Build history of the part. All positions in model axes, mm. A direction names the side the tool comes from. Give positions to 0.01 mm unless a question says otherwise; leave off trailing zeros. Write each loop counter-clockwise with the first axis right and the second up, starting at its lowest first coordinate (ties: lowest second). Pieces come first, ordered by that corner, then holes. Notation, with made-up numbers: (43, -24.75) - (77, -24.75) arc R22 ccw to (77, -18.75) - close; hole circle Ø7 at (27, 63). An arc over 180 degrees is marked (long way). Use one line per item in the form item = value. Start each with the question number.
from build123d import *

# Parameters (mm, degrees)
BOSS_EXTRUDE1_DEPTH     = 25.4
SKETCH2_W               = 52
SKETCH2_H               = 63.5
CUT_EXTRUDE1_DEPTH      = 3.175
SKETCH3_W               = 25.4
SKETCH3_H               = 63.5
CUT_EXTRUDE2_DEPTH      = 3.175
SKETCH4_W               = 52
SKETCH4_H               = 63.5
CUT_EXTRUDE3_DEPTH      = 3.175
SKETCH5_W               = 25.4
SKETCH5_H               = 63.5
CUT_EXTRUDE4_DEPTH      = 3.175
SKETCH6_R               = 2.5527
CUT_EXTRUDE5_DEPTH      = 23.225
SKETCH7_R               = 2.5527
CUT_EXTRUDE6_DEPTH      = 150.825
SKETCH8_W               = 101
SKETCH8_H               = 177.8
CUT_EXTRUDE7_DEPTH      = 26.4
CUT_EXTRUDE8_DEPTH      = 1
CUT_EXTRUDE8_DEPTH_BACK = 26.4
CUT_EXTRUDE9_DEPTH      = 26.4
CUT_EXTRUDE10_DEPTH     = 26.4
BOSS_EXTRUDE2_DEPTH     = 25.4
CUT_EXTRUDE11_DEPTH     = 51.8
CUT_EXTRUDE12_DEPTH     = 51.8
CUT_EXTRUDE13_DEPTH     = 93.323036631
CUT_EXTRUDE14_DEPTH     = 51.8
CUT_EXTRUDE15_DEPTH     = 26.4
CUT_EXTRUDE16_DEPTH     = 51.8


with BuildPart() as part:
    # Sketch1 → Boss-Extrude1 (new body)
    with BuildSketch(Plane.XY):
        Polygon((0, 0), (0, 76.2), (-101, 76.2), (-101, 254), (153, 254), (153, 76.2), (52, 76.2), (52, 0), align=None)
    extrude(amount=BOSS_EXTRUDE1_DEPTH)

    # Sketch2 → Cut-Extrude1 (cut)
    with BuildSketch(Plane.XY.offset(25.4)):
        with Locations((26, 31.75)):
            Rectangle(SKETCH2_W, SKETCH2_H)
    extrude(amount=-CUT_EXTRUDE1_DEPTH, mode=Mode.SUBTRACT)

    # Sketch3 → Cut-Extrude2 (cut)
    with BuildSketch(Plane.ZY):
        with Locations((12.7, 31.75)):
            Rectangle(SKETCH3_W, SKETCH3_H)
    extrude(amount=-CUT_EXTRUDE2_DEPTH, mode=Mode.SUBTRACT)

    # Sketch4 → Cut-Extrude3 (cut)
    with BuildSketch(Plane(origin=(0, 0, 0), x_dir=(-1, 0, 0), z_dir=(0, 0, -1))):
        with Locations((-26, 31.75)):
            Rectangle(SKETCH4_W, SKETCH4_H)
    extrude(amount=-CUT_EXTRUDE3_DEPTH, mode=Mode.SUBTRACT)

    # Sketch5 → Cut-Extrude4 (cut)
    with BuildSketch(Plane(origin=(52, 0, 0), x_dir=(0, 0, -1), z_dir=(1, 0, 0))):
        with Locations((-12.7, 31.75)):
            Rectangle(SKETCH5_W, SKETCH5_H)
    extrude(amount=-CUT_EXTRUDE4_DEPTH, mode=Mode.SUBTRACT)

    # Sketch6 → Cut-Extrude5 (cut, through all)
    with BuildSketch(Plane(origin=(0, 0, 3.175), x_dir=(-1, 0, 0), z_dir=(0, 0, -1))):
        with Locations((-39.3, 57.15)):
            Circle(SKETCH6_R)
        with Locations((-13.9, 57.15)):
            Circle(SKETCH6_R)
        with Locations((-39.3, 44.45)):
            Circle(SKETCH6_R)
        with Locations((-13.9, 44.45)):
            Circle(SKETCH6_R)
        with Locations((-39.3, 31.75)):
            Circle(SKETCH6_R)
        with Locations((-13.9, 31.75)):
            Circle(SKETCH6_R)
        with Locations((-39.3, 19.05)):
            Circle(SKETCH6_R)
        with Locations((-13.9, 19.05)):
            Circle(SKETCH6_R)
        with Locations((-39.3, 6.35)):
            Circle(SKETCH6_R)
        with Locations((-13.9, 6.35)):
            Circle(SKETCH6_R)
    extrude(amount=-CUT_EXTRUDE5_DEPTH, mode=Mode.SUBTRACT)

    # Sketch7 → Cut-Extrude6 (cut, through all)
    with BuildSketch(Plane(origin=(48.825, 0, 0), x_dir=(0, 0, -1), z_dir=(1, 0, 0))):
        with Locations((-12.7, 57.15)):
            Circle(SKETCH7_R)
        with Locations((-12.7, 44.45)):
            Circle(SKETCH7_R)
        with Locations((-12.7, 31.75)):
            Circle(SKETCH7_R)
        with Locations((-12.7, 19.05)):
            Circle(SKETCH7_R)
        with Locations((-12.7, 6.35)):
            Circle(SKETCH7_R)
    extrude(amount=-CUT_EXTRUDE6_DEPTH, mode=Mode.SUBTRACT)

    # Sketch8 → Cut-Extrude7 (cut, through all)
    with BuildSketch(Plane.XY.offset(25.4)):
        with Locations((102.5, 165.1)):
            Rectangle(SKETCH8_W, SKETCH8_H)
    extrude(amount=-CUT_EXTRUDE7_DEPTH, mode=Mode.SUBTRACT)

    # Sketch9 → Cut-Extrude8 (cut, two sides)
    with BuildSketch(Plane.XY.offset(25.4)) as cut_extrude8_sk:
        Polygon((52, 254), (52, 242.697), (35.85764308, 254), align=None)
    extrude(amount=CUT_EXTRUDE8_DEPTH, mode=Mode.SUBTRACT)
    extrude(cut_extrude8_sk.sketch, amount=-CUT_EXTRUDE8_DEPTH_BACK, mode=Mode.SUBTRACT)

    # Sketch10 → Cut-Extrude9 (cut, through all)
    with BuildSketch(Plane.XY.offset(25.4)):
        Polygon((35.85764308, 254), (-101, 58.547029828), (-101, 254), align=None)
    extrude(amount=-CUT_EXTRUDE9_DEPTH, mode=Mode.SUBTRACT)

    # Sketch11 → Cut-Extrude10 (cut, through all)
    with BuildSketch(Plane.XY.offset(25.4)):
        Polygon((35.85764308, 254), (46.79768076, 246.339703148), (-82.829822213, 61.212443159), (-93.769859893, 68.872740011), align=None)
    extrude(amount=-CUT_EXTRUDE10_DEPTH, mode=Mode.SUBTRACT)

    # Sketch14 → Boss-Extrude2 (add)
    with BuildSketch(Plane.XY.offset(25.4)):
        Polygon((46.79768076, 246.339703148), (69.685492552, 230.313484798), (-62.703014112, 41.243102891), (-85.590825904, 57.26932124), align=None)
    extrude(amount=BOSS_EXTRUDE2_DEPTH)

    # Sketch15 → Cut-Extrude11 (cut, through all)
    with BuildSketch(Plane.XY.offset(50.8)):
        Polygon((-38.225931244, 76.2), (-72.335421933, 76.2), (-85.590825904, 57.26932124), (-62.703014112, 41.243102891), align=None)
    extrude(amount=-CUT_EXTRUDE11_DEPTH, mode=Mode.SUBTRACT)

    # Sketch16 → Cut-Extrude12 (cut, through all)
    with BuildSketch(Plane(origin=(0, 0, 0), x_dir=(-1, 0, 0), z_dir=(0, 0, -1))):
        Polygon((0, 76.2), (40.323036631, 121.918424261), (72.335421933, 76.2), align=None)
    extrude(amount=-CUT_EXTRUDE12_DEPTH, mode=Mode.SUBTRACT)

    # Sketch17 → Cut-Extrude13 (cut, through all)
    with BuildSketch(Plane(origin=(52, 0, 0), x_dir=(0, 0, -1), z_dir=(1, 0, 0))):
        Polygon((-12.7, 246.339703148), (-12.7, 100.289703148), (0, 76.2), (0, 246.339703148), align=None)
    extrude(amount=-CUT_EXTRUDE13_DEPTH, mode=Mode.SUBTRACT)

    # Sketch18 → Cut-Extrude14 (cut, through all)
    with BuildSketch(Plane.XY.offset(50.8)):
        Polygon((64.483173396, 233.956187887), (-27.012035852, 103.287487173), (-44.697528488, 115.671002434), (46.79768076, 246.339703148), align=None)
    extrude(amount=-CUT_EXTRUDE14_DEPTH, mode=Mode.SUBTRACT)

    # Sketch19 → Cut-Extrude15 (cut, through all)
    with BuildSketch(Plane(origin=(0, 0, 25.4), x_dir=(-1, 0, 0), z_dir=(0, 0, -1))):
        Polygon((-52, 205.055983862), (-52, 216.128368684), (-64.483173396, 233.956187887), (-69.685492552, 230.313484798), align=None)
    extrude(amount=-CUT_EXTRUDE15_DEPTH, mode=Mode.SUBTRACT)

    # Sketch20 → Cut-Extrude16 (cut, through all)
    with BuildSketch(Plane.XY.offset(50.8)):
        Polygon((52, 205.055983862), (46.797680844, 208.698686951), (52, 216.128368684), align=None)
    extrude(amount=-CUT_EXTRUDE16_DEPTH, mode=Mode.SUBTRACT)


solid = part.part
(1) Cut at A-A, the plane y = 57.15. Give the cut face in (x, z) (3 decimals).
(2) Two-plate mould, pull along X, no slides. Class faces 3 (the flat face through (24, 120, 25.4)), 4 (the cylindrical face through (11.542, 5.372, 6.812)), 5 (the flat face through (49.44, 206.85, 32.02)): +X half, -X half, draft (parallel to the pull), parting line (faces both ways), or undercut.
(3) Cut at D-D, the plane y = 80. Give the cut face in (x, z), then the cut area to 3 significant figures.
(4) Cut at B-B, the plane z = 5.5. State how many separate pieces and enclosed holes the cut face has, then the cut area to 3 significant figures.
(5) Wall check: line 1 (X direction, y = 6, z = 9) (3 decimals); line 2 (X direction, y = 6.35, z = 16.5) (3 decimals); line 3 (Y direction, x = 13, z = 17). Give the ranges that are in metal, low to high. Write a range as from..to.
(6) Pin check, flat tips, straight feed: pin 1 Ø1.5 at (x, y) = (18, 79.5) entering from +Z; pin 2 Ø6.5 at (x, y) = (13.9, 44.45) entering from +Z (3 decimals); pin 3 Ø13.5 at (x, y) = (28.5, 25.5) entering from -Z (3 decimals); pin 4 Ø6 at (x, z) = (36.5, 6.5) entering from -Y. Stop position of each tip, or through.
(7) Cut at C-C, the plane z = 47. Give the cut face in (x, y), then the cut area to 3 significant figures.
(8) Which spindle directions (+Z, -Z, +X, -X, +Y, -Y) get a long thin tool onto all of the face, cutting with end or side? Do faces 1 (the flat face through (15.86, 153.44, 37.92)), 2 (the cylindrical face through (7.421, 59.302, 11.328)). Say none if no direction does.
Solution:
q1.outline = (3.175, 3.175) - (11.347, 3.175) - (11.347, 10.147) - (3.175, 10.147) - close; (3.175, 15.253) - (11.347, 15.253) - (11.347, 22.225) - (3.175, 22.225) - close; (16.453, 3.175) - (36.747, 3.175) - (36.747, 10.147) - (16.453, 10.147) - close; (16.453, 15.253) - (36.747, 15.253) - (36.747, 22.225) - (16.453, 22.225) - close; (41.853, 3.175) - (48.825, 3.175) - (48.825, 10.147) - (41.853, 10.147) - close; (41.853, 15.253) - (48.825, 15.253) - (48.825, 22.225) - (41.853, 22.225) - close
q2.face_3 = draft
q2.face_4 = undercut
q2.face_5 = +X half
q3.outline = (-3.35, 2) - (52, 2) - (52, 25.4) - (-3.35, 25.4) - close
q3.area = 1,300 mm2
q4.separate_pieces = 1
q4.enclosed_holes = 10
q4.area = 3,940 mm2
q5.line_1 = 3.175..11.371, 16.429..36.771, 41.829..48.825
q5.line_2 = 3.175..11.347, 16.453..36.747, 41.853..48.825
q5.line_3 = 0..3.96, 8.74..16.66, 21.44..29.36, 34.14..42.06, 46.84..54.76, 59.54..160.43
q6.pin_1 = 25.4
q6.pin_2 = 22.225
q6.pin_3 = 3.175
q6.pin_4 = 0
q7.outline = (-25.63, 105.26) - (-21.31, 100.36) - (52, 205.06) - (46.8, 208.7) - close
q7.area = 807 mm2
q8.face_1 = +Z, +X, -Y
q8.face_2 = +X, -X
